```python
from build123d import *

# Parameters (mm, degrees)
CYLINDER018_R          = 1.6
CYLINDER018_DEPTH      = 1
CYLINDER017_R          = 4.5
CYLINDER017_DEPTH      = 1
CUT020_PLACEMENT_ANGLE = 90


with BuildPart() as facewasherscrewhole:
    # Cylinder018 → Cylinder018 (new body)
    with BuildSketch(Plane.XY):
        Circle(CYLINDER018_R)
    extrude(amount=CYLINDER018_DEPTH)


with BuildPart() as facewasher001:
    # Cylinder017 → Cylinder017 (new body)
    with BuildSketch(Plane.XY):
        Circle(CYLINDER017_R)
    extrude(amount=CYLINDER017_DEPTH)

    # Cut020: cut FaceWasherScrewHole
    add(facewasherscrewhole.part, mode=Mode.SUBTRACT)


with BuildPart() as facewasher001_1:
    # Cut020 placement: moved
    add(facewasher001.part.moved(Location((0, 0, -1))).rotate(Axis((0, 0, -1), (1, 0, 0)), CUT020_PLACEMENT_ANGLE))


with BuildPart() as facewasher001_2:
    # Clone021 placement: moved
    add(facewasher001_1.part.moved(Location((-8.5, 3, 8))))


with BuildPart() as part_mirroring023:
    # Part__Mirroring023: instance of FaceWasher001
    add(facewasher001_2.part.mirror(Plane(origin=(87, 0, 0), x_dir=(0, -1, 0), z_dir=(1, 0, 0))))


solid = part_mirroring023.part
```
Model file for the job. Use its own axes, mm. Coordinates: 2 decimals unless noted, no trailing zeros. Write each loop counter-clockwise with the first axis right and the second up, starting at its lowest first coordinate (ties: lowest second). Pieces come first, ordered by that corner, then holes. Notation, with made-up numbers: (77, 9.25) - (93, 9.25) arc R17 ccw to (93, 17.25) - close; hole circle Ø1 at (73, 64.5). An arc over 180 degrees is marked (long way). One line per question, with ' | ' between items. Start each with the question number.
Q1. Drill centre lines: line 1 (Z direction, x = 182.5, y = 2.4); line 2 (Z direction, x = 183.25, y = 2.9); line 3 (X direction, y = 2.4, z = 6.25). Where is each one in solid material? Low to high. Write a range as [from, to].
Q2. Cut at A-A, the plane x = 182.5. List the corners of the cut face in (y, z).
Q3. Pin check, flat tip, straight feed: pin 1 (2.5 mm diameter, centred on x = 182.5, z = 7, fed in from +Y). Stop position of the tip, or through.
Q4. Cut at B-B, the plane z = 7. List the corners of the cut face in (x, y), then the cut area to 3 significant figures.
Q5. Cut at C-C, the plane y = 2.8. List the corners of the cut face in (x, z).
Q6. Cut at D-D, the plane z = 9.75. List the corners of the cut face in (x, y).
Answer below:
1) line 1: [2.5, 5.4], [8.6, 11.5] | line 2: [2.56, 5.59], [8.41, 11.44] | line 3: [178.06, 181.09], [183.91, 186.94]
2) outline: (2, 2.5) - (3, 2.5) - (3, 5.4) - (2, 5.4) - close; (2, 8.6) - (3, 8.6) - (3, 11.5) - (2, 11.5) - close
3) pin 1: through
4) outline: (178, 2) - (180.9, 2) - (180.9, 3) - (178, 3) - close; (184.1, 2) - (187, 2) - (187, 3) - (184.1, 3) - close | area: 5.80 mm^2
5) outline: circle Ø9 at (182.5, 7); hole circle Ø3.2 at (182.5, 7)
6) outline: (178.94, 2) - (186.06, 2) - (186.06, 3) - (178.94, 3) - close
